The model under review builds one solid part; all positions refer to its coordinate system, in mm. Round coordinates to 2 decimals unless told otherwise and drop trailing zeros. Write each loop counter-clockwise with the first axis right and the second up, starting at its lowest first coordinate (ties: lowest second). Pieces come first, ordered by that corner, then holes. Notation, with made-up numbers: (47.25, 29) -> (56.25, 29) arc R17 cw to (56.25, 57) -> close; hole circle Ø3 at (-28.5, -22). An arc over 180 degrees is marked (long way). Return JSON: item names as keys, results as strings. Group by question number.
1. Mouldability with a two-part tool opening along Z and no side actions: class faces 1 (the flat face through (0, 10, 1)), 2 (the flat face through (0, 5, -92.5)), 3 (the cylindrical face through (0.56, 4.93, 0.04)) as pulls with the +Z half, pulls with the -Z half, needs draft (parallel to the pull), parting line crosses it, or undercut.
2. Take a section at A-A, the plane z = -42.5. Write out the cut boundary in (x, y).
3. For line 1 along X through (y, z) = (4.5, 17); line 2 along X through (y, z) = (4.5, 55.5), list the stretches that pass through material, from the lowest coordinate up. Write a range as from..to.
4. Clearance check with a flat-ended pin moving along its axis: P1, Ø3, axis at x = 0, z = -22.5, coming from the +Y side. State where the tip first meets the part, or that it passes through.
5. Take a section at B-B, the plane y = 7.25. Give the number of separate pieces and of enclosed holes in the cut face, then the cut area to 3 significant figures.
Autodesk Inventor part; units mm, degrees
ref_plane "YZ Plane" through (0, 0, 0) normal (1, 0, 0) x (0, 1, 0)
ref_plane "XZ Plane" through (0, 0, 0) normal (0, 1, 0) x (-1, 0, 0)
ref_plane "XY Plane" through (0, 0, 0) normal (0, 0, 1) x (1, 0, 0)
sketch "Sketch1" plane through (0, 0, 0) normal (0, 1, 0) x (-1, 0, 0)
  line L0 (-10, 92.5) -> (10, 92.5)
  line L1 (10, 92.5) -> (10, -92.5)
  line L2 (10, -92.5) -> (-10, -92.5)
  line L3 (-10, -92.5) -> (-10, 92.5)
  line L4 (-10, 92.5) -> (10, -92.5) construction
  line L5 (10, 92.5) -> (-10, -92.5) construction
  circle A0 centre (0, -82.5) radius 2.6
  circle A1 centre (0, -72.5) radius 2.6
  circle A2 centre (0, -62.5) radius 2.6
  circle A3 centre (0, -52.5) radius 2.6
  circle A4 centre (0, -42.5) radius 2.6
  circle A5 centre (0, -32.5) radius 2.6
  circle A6 centre (0, -22.5) radius 2.6
  circle A7 centre (0, -12.5) radius 2.6
  circle A8 centre (0, -2.5) radius 2.6
  circle A9 centre (0, 7.5) radius 2.6
  circle A10 centre (0, 17.5) radius 2.6
  circle A11 centre (0, 27.5) radius 2.6
  circle A12 centre (0, 37.5) radius 2.6
  circle A13 centre (0, 47.5) radius 2.6
  circle A14 centre (0, 57.5) radius 2.6
  circle A15 centre (0, 67.5) radius 2.6
  circle A16 centre (0, 77.5) radius 2.6
  circle A17 centre (0, 87.5) radius 2.6
  circle A18 centre (0, 97.5) radius 2.6
  circle A19 centre (0, 107.5) radius 2.6
  circle A20 centre (0, 117.5) radius 2.6
  circle A21 centre (0, 127.5) radius 2.6
  circle A22 centre (0, 137.5) radius 2.6
  circle A23 centre (0, 147.5) radius 2.6
  point P0 (0, 0)
  dimension "d0" = 20
  dimension "d1" = 185
  dimension "d2" = 10
  dimension "d3" = 5.2
  dimension "d6" = 10
extrude "Extrusion1" add sketch "Sketch1" along normal blind 10 contours L0 L1 L2 L3
properties part number "Zarm" material "Wood (Birch)"
Output:
{
 "1": {"face 1": "needs draft", "face 2": "pulls with the -Z half", "face 3": "undercut"},
 "2": {"outline": "(-10, 0) -> (-2.6, 0) -> (-2.6, 10) -> (-10, 10) -> close; (2.6, 0) -> (10, 0) -> (10, 10) -> (2.6, 10) -> close"},
 "3": {"line 1": "x = -10..-2.55, 2.55..10", "line 2": "x = -10..-1.66, 1.66..10"},
 "4": {"P1": "passes through"},
 "5": {"separate pieces": "1", "enclosed holes": "18", "area": "3,320 mm^2"}
}
